For this review, take the finished solid that the model builds, in its own axes (mm). Face numbers are marked on the shaded views. A direction names the side the tool comes from. Round coordinates to 2 decimals unless told otherwise and drop trailing zeros. Loops run counter-clockwise (first coordinate to the right, second up) from the corner with the lowest first, then second, coordinate; pieces in that order, holes last.
1. Consider section B-B on y = 8. State the section outline as (x, z) points, then the cut area to 3 significant figures.
2. Clearance check with flat-ended pins moving along their axes: pin 1 Ø2 at (x, y) = (-18, 17.5) entering from -Z; pin 2 Ø6 at (y, z) = (21, -19) entering from -X; pin 3 Ø2 at (y, z) = (19.5, -12) entering from +X. State where each tip first meets the part, or that it passes through.
3. Tool access review of the marked faces 4 and 5: name each direction out of +Z, -Z, +X, -X, +Y, -Y from which nothing blocks a thin tool from reaching the whole face with its end or side.
4. Draft analysis for pull direction Y (two halves, no side actions). For the marked faces 1, 2 and 3, state which applies: released by +Y, released by -Y, zero draft, split by the parting line, or undercut.
5. To check wall thickness, follow line 1 along X through (y, z) = (3.5, -12); line 2 along X through (y, z) = (17.5, -13); line 3 along Z through (x, y) = (0.5, 35.5). State the ranges of each line that lie inside material, in increasing order.
6. Consider section A-A on x = 0. State the section outline as (y, z) points.
7. Consider section C-C on y = 32. State the section outline as (x, z) points, then the cut area to 3 significant figures.
from build123d import *

# Parameters (mm, degrees)
CUT_EXTRUDE3_DEPTH           = 25
CUT_EXTRUDE3_DEPTH_BACK      = 40
CUT_EXTRUDE5_START           = -5
CUT_EXTRUDE5_DEPTH           = 5
BOSS_EXTRUDE2_DEPTH          = 5
SKETCH14_R                   = 1
BOSS_EXTRUDE3_DEPTH          = 3
BOSS_EXTRUDE4_START          = 3
SKETCH15_R                   = 1
BOSS_EXTRUDE4_DEPTH          = 3
CUT_EXTRUDE6_DEPTH           = 22
SKETCH17_W                   = 7
SKETCH17_H                   = 20.303986046
CUT_REVOLVE1_ANGLE           = 45
CUT_REVOLVE1_OTHER_WAY_ANGLE = 45
INTERSECT1_OUTLINE_W         = 62
INTERSECT1_OUTLINE_H         = 54
INTERSECT1_DEPTH             = 31
INTERSECT1_START             = -5
INTERSECT1_2_OUTLINE_W       = 12
INTERSECT1_2_OUTLINE_H       = 4
INTERSECT1_2_DEPTH           = 5


with BuildPart() as part:
    # Sketch1 → Revolve1 (revolve)
    with BuildSketch(Plane.XY, mode=Mode.PRIVATE) as revolve1_sk:
        with BuildLine():
            Line((20.9, 0), (23.871591838, 0))
            Line((23.871591838, 0), (23.871591838, 4))
            Line((23.871591838, 4), (22.9, 4.236662843))
            Line((22.9, 4.236662843), (22.9, 11.874576818))
            ThreePointArc((22.9, 11.874576818), (23.83692213, 16.100759435), (26.472123903, 19.535021249))
            Line((26.472123903, 19.535021249), (26.427876097, 19.497892931))
            ThreePointArc((26.427876097, 19.497892931), (29.06307787, 22.932154745), (30, 27.158337362))
            Line((30, 27.158337362), (30, 50))
            ThreePointArc((30, 50), (28.828427125, 52.828427125), (26, 54))
            Line((26, 54), (0, 54))
            Line((0, 54), (0, 15))
            Line((0, 15), (19.9, 15))
            ThreePointArc((19.9, 15), (20.607106781, 14.707106781), (20.9, 14))
            Line((20.9, 14), (20.9, 0))
        make_face()
    revolve(revolve1_sk.sketch.rotate(Axis((0, 0, 0), (0, 1, 0)), 90), axis=Axis((0, 0, 0), (0, 1, 0)))

    # Sketch11 → Cut-Extrude3 (cut, two sides: drawn at the far end of the back side and taken through both)
    with BuildSketch(Plane(origin=(0, 19.535021249, 0), x_dir=(-1, 0, 0), z_dir=(0, -1, 0)).offset(-CUT_EXTRUDE3_DEPTH_BACK)):
        with BuildLine():
            Line((-17.5, 0), (17.5, 0))
            ThreePointArc((17.5, 0), (0, 17.5), (-17.5, 0))
        make_face()
    extrude(amount=CUT_EXTRUDE3_DEPTH + CUT_EXTRUDE3_DEPTH_BACK, mode=Mode.SUBTRACT)

    # Sketch9 → Cut-Extrude5 (cut)
    with BuildSketch(Plane(origin=(0, 50, 0), x_dir=(-1, 0, 0), z_dir=(0, -1, 0)).offset(CUT_EXTRUDE5_START)):
        with BuildLine():
            Line((-30, 0), (30, 0))
            ThreePointArc((30, 0), (0, 30), (-30, 0))
        make_face()
    extrude(amount=CUT_EXTRUDE5_DEPTH, mode=Mode.SUBTRACT)

    # Sketch13 → Boss-Extrude2 (add)
    with BuildSketch(Plane(origin=(0, 0, 0), x_dir=(-1, 0, 0), z_dir=(0, 0, -1))):
        with BuildLine():
            Line((22.5, 53.5), (26.5, 53.5))
            ThreePointArc((26.5, 53.5), (26.853553391, 53.353553391), (27, 53))
            Line((27, 53), (27, 51))
            ThreePointArc((27, 51), (26.853553391, 50.646446609), (26.5, 50.5))
            Line((26.5, 50.5), (22.5, 50.5))
            ThreePointArc((22.5, 50.5), (22.146446609, 50.646446609), (22, 51))
            Line((22, 51), (22, 53))
            ThreePointArc((22, 53), (22.146446609, 53.353553391), (22.5, 53.5))
        make_face()
        with BuildLine():
            Line((-26.5, 53.5), (-22.5, 53.5))
            ThreePointArc((-22.5, 53.5), (-22.146446609, 53.353553391), (-22, 53))
            Line((-22, 53), (-22, 51))
            ThreePointArc((-22, 51), (-22.146446609, 50.646446609), (-22.5, 50.5))
            Line((-22.5, 50.5), (-26.5, 50.5))
            ThreePointArc((-26.5, 50.5), (-26.853553391, 50.646446609), (-27, 51))
            Line((-27, 51), (-27, 53))
            ThreePointArc((-27, 53), (-26.853553391, 53.353553391), (-26.5, 53.5))
        make_face()
    extrude(amount=BOSS_EXTRUDE2_DEPTH)

    # Sketch14 → Boss-Extrude3 (add)
    with BuildSketch(Plane.ZY.offset(-22)):
        with Locations(Location((-3, 52, 0), (0, 0, 270))):
            Circle(SKETCH14_R)
    extrude(amount=BOSS_EXTRUDE3_DEPTH)

    # Sketch15 → Boss-Extrude4 (add)
    with BuildSketch(Plane(origin=(-22, 0, 0), x_dir=(0, 0, -1), z_dir=(1, 0, 0)).offset(BOSS_EXTRUDE4_START)):
        with Locations(Location((3, 52, 0), (0, 0, 270))):
            Circle(SKETCH15_R)
    extrude(amount=-BOSS_EXTRUDE4_DEPTH)

    # Sketch16 → Cut-Extrude6 (cut)
    with BuildSketch(Plane(origin=(0, 50, 0), x_dir=(-1, 0, 0), z_dir=(0, -1, 0))):
        with BuildLine():
            Line((25.690465157, -4), (-25.690465157, -4))
            ThreePointArc((-25.690465157, -4), (0, -26), (25.690465157, -4))
        make_face()
    extrude(amount=CUT_EXTRUDE6_DEPTH, mode=Mode.SUBTRACT)

    # Sketch17 → Cut-Revolve1 (revolve, cut)
    with BuildSketch(Plane(origin=(0, 0, 0), x_dir=(0, 0, -1), z_dir=(1, 0, 0))):
        with Locations((-28.883918314, 38.580330385)):
            Rectangle(SKETCH17_W, SKETCH17_H)
    revolve(axis=Axis((0, 0, 0), (0, 0.9999633813881498, 0.008557796607647805)), revolution_arc=CUT_REVOLVE1_ANGLE, mode=Mode.SUBTRACT)

    # Sketch17 → Cut-Revolve1 other way (revolve, cut)
    with BuildSketch(Plane(origin=(0, 0, 0), x_dir=(0, 0, -1), z_dir=(1, 0, 0))):
        with Locations((-28.883918314, 38.580330385)):
            Rectangle(SKETCH17_W, SKETCH17_H)
    revolve(axis=Axis((0, 0, 0), (0, -0.9999633813881498, -0.008557796607647805)), revolution_arc=CUT_REVOLVE1_OTHER_WAY_ANGLE, mode=Mode.SUBTRACT)

    # Intersect1: read off the stored shape, not the designer's step
    # Intersect1 outline → Intersect1 (cut)
    with BuildSketch(Plane.XY):
        with Locations((0, 27)):
            Rectangle(INTERSECT1_OUTLINE_W, INTERSECT1_OUTLINE_H)
    extrude(amount=INTERSECT1_DEPTH, mode=Mode.SUBTRACT)

    # Intersect1 2 outline → Intersect1 2 (cut)
    with BuildSketch(Plane.XY.offset(INTERSECT1_START)):
        with Locations((-25, 52)):
            Rectangle(INTERSECT1_2_OUTLINE_W, INTERSECT1_2_OUTLINE_H)
        with Locations((25, 52)):
            Rectangle(INTERSECT1_2_OUTLINE_W, INTERSECT1_2_OUTLINE_H)
    extrude(amount=INTERSECT1_2_DEPTH, mode=Mode.SUBTRACT)


solid = part.part
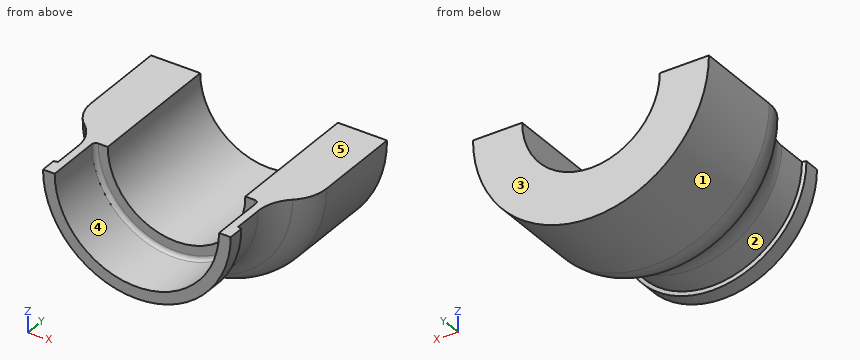
Resolved:
1. outline: (-22.9, 0) arc R22.9 ccw to (22.9, 0) - (20.9, 0) arc R20.9 cw to (-20.9, 0) - close
1. area: 138 mm2
2. pin 1: stops at z = -18.28
2. pin 2: stops at x = -23.78
2. pin 3: stops at x = 24.81
3. face 4: +Z, -Y
3. face 5: +Z, +X, -X, +Y, -Y
4. face 1: zero draft
4. face 2: undercut
4. face 3: released by +Y
5. line 1: x = -20.64 to -17.11, 17.11 to 20.64
5. line 2: x = -20.92 to -11.72, 11.72 to 20.92
5. line 3: z = -30 to -17.49
6. outline: (0, -23.87) - (4, -23.87) - (4.24, -22.9) - (11.87, -22.9) arc R10 cw to (19.54, -26.47) - (19.5, -26.43) arc R10 ccw to (27.16, -30) - (50, -30) - (50, -17.5) - (15, -17.5) - (15, -19.9) arc R1 cw to (14, -20.9) - (0, -20.9) - close
7. outline: (-30, 0) arc R30 ccw to (30, 0) - (17.5, 0) arc R17.5 cw to (-17.5, 0) - close
7. area: 933 mm2
